For this review, take the finished solid that the model builds, in its own axes (mm). A direction names the side the tool comes from. Round coordinates to 2 decimals unless told otherwise and drop trailing zeros. Loops run counter-clockwise (first coordinate to the right, second up) from the corner with the lowest first, then second, coordinate; pieces in that order, holes last. Notation, with made-up numbers: M 8,64.25 L 59,64.25 A33 cw 59,99.25 Z; hole C 65.25,-1.5 d5. An arc over 180 degrees is marked long. Write item = value, one per line. Start each with the question number.
```python
from build123d import *

# Parameters (mm, degrees)
F0_W     = 82.55
F0_H     = 57.15
F0_W_2   = 76.2
F0_H_2   = 50.8
F1_DEPTH = 25.4
F2_W     = 19.05
F2_H     = 19.05
F3_DEPTH = 22.86


with BuildPart() as f1:
    # F0 (on Front) → F1 (new body)
    with BuildSketch(Plane.XZ):
        Rectangle(F0_W, F0_H)
        Rectangle(F0_W_2, F0_H_2, mode=Mode.SUBTRACT)
        Rectangle(F0_W_2, F0_H_2)
    extrude(amount=F1_DEPTH)

    # F2 (on Front) → F3 (cut)
    with BuildSketch(Plane.XZ):
        with Locations((26.126538, 15.033415)):
            Rectangle(F2_W, F2_H)
        with Locations((0, 15.033415)):
            Rectangle(F2_W, F2_H)
        with Locations((-29.117243, 15.033415)):
            Rectangle(F2_W, F2_H)
        with Locations((-27.96792, -17.036804)):
            Rectangle(F2_W, F2_H)
        with Locations((0, -17.552111)):
            Rectangle(F2_W, F2_H)
        with Locations((26.873696, -17.036807)):
            Rectangle(F2_W, F2_H)
    extrude(amount=F3_DEPTH, mode=Mode.SUBTRACT)


solid = f1.part
```
(1) Draft analysis for pull direction Z (two halves, no side actions). For faces 3 (the flat face through (-1, -13, 28.575)), 4 (the flat face through (-41.275, -13, 0)), 5 (the flat face through (27, -22.86, -17)), state which applies: +Z half, -Z half, draft (parallel to the pull), parting line (faces both ways), or undercut.
(2) Add section B-B on z = 12.5. Write out the cut boundary in (x, y) (3 decimals), and give its area (3 significant figures).
(3) Add section C-C on x = 31. Write out the cut boundary in (y, z) (3 decimals), and give its area (3 significant figures).
(4) Add section A-A on y = -5.5. Write out the cut boundary in (x, z) (3 decimals), and give its area (3 significant figures).
(5) For pin 1 Ø1 at (x, z) = (-24, 5.5) entering from +Y, flat-tipped, find the tip position at first contact; note if it passes through.
(6) Wall thickness on L1, parallel to X at y = -2, z = -24 (3 decimals); L2, parallel to Z at x = -29.5, y = -13.75 (3 decimals); L3, parallel to X at y = -12.25, z = 7 (3 decimals): over which ranges is each line inside the solid? List them lowest first.
(7) Tool access review of faces 1 (the flat face through (16.602, -11, 15)), 2 (the flat face through (-1, -13, -28.575)): name each direction out of +Z, -Z, +X, -X, +Y, -Y from which nothing blocks a thin tool from reaching the whole face with its end or side.
Answer sheet:
q1.face_3 = +Z half
q1.face_4 = draft
q1.face_5 = undercut
q2.outline = M -41.275,-25.4 L 41.275,-25.4 L 41.275,0 L 35.652,0 L 35.652,-22.86 L 16.602,-22.86 L 16.602,0 L 9.525,0 L 9.525,-22.86 L -9.525,-22.86 L -9.525,0 L -19.592,0 L -19.592,-22.86 L -38.642,-22.86 L -38.642,0 L -41.275,0 Z
q2.area = 790 mm²
q3.outline = M -25.4,-28.575 L 0,-28.575 L 0,-26.562 L -22.86,-26.562 L -22.86,-7.512 L 0,-7.512 L 0,5.508 L -22.86,5.508 L -22.86,24.558 L 0,24.558 L 0,28.575 L -25.4,28.575 Z
q3.area = 581 mm²
q4.outline = M -41.275,-28.575 L 41.275,-28.575 L 41.275,28.575 L -41.275,28.575 Z; hole M -38.642,5.508 L -19.592,5.508 L -19.592,24.558 L -38.642,24.558 Z; hole M -37.493,-26.562 L -18.443,-26.562 L -18.443,-7.512 L -37.493,-7.512 Z; hole M -9.525,-27.077 L 9.525,-27.077 L 9.525,-8.027 L -9.525,-8.027 Z; hole M -9.525,5.508 L 9.525,5.508 L 9.525,24.558 L -9.525,24.558 Z; hole M 16.602,5.508 L 35.652,5.508 L 35.652,24.558 L 16.602,24.558 Z; hole M 17.349,-26.562 L 36.399,-26.562 L 36.399,-7.512 L 17.349,-7.512 Z
q4.area = 2,540 mm²
q5.pin_1 = 0
q6.L1 = -41.275 to -37.493, -18.443 to -9.525, 9.525 to 17.349, 36.399 to 41.275
q6.L2 = -28.575 to -26.562, -7.512 to 5.508, 24.558 to 28.575
q6.L3 = -41.275 to -38.642, -19.592 to -9.525, 9.525 to 16.602, 35.652 to 41.275
q7.face_1 = +Y
q7.face_2 = -Z, +X, -X, +Y, -Y
